Geometry: final body of the model. Coordinates: model frame, mm. Face numbers are marked on the shaded views. A direction names the side the tool comes from. Give positions to 0.01 mm unless a question says otherwise; leave off trailing zeros. Loops run counter-clockwise (first coordinate to the right, second up) from the corner with the lowest first, then second, coordinate; pieces in that order, holes last. Notation, with made-up numbers: (44.5, 19) - (80.5, 19) arc R29 cw to (80.5, 50) - close; hole circle Ø10 at (-12, 51.25). An arc over 180 degrees is marked (long way). Answer in a Markdown table with one row per item.
from build123d import *

# Parameters (mm, degrees)
BOSS_EXTRUDE1_DEPTH     = 10
CUT_EXTRUDE2_DEPTH      = 45.988887517
CUT_EXTRUDE2_DEPTH_BACK = 45.988887517
SKETCH5_R               = 2
CUT_EXTRUDE3_DEPTH      = 44.874821937


with BuildPart() as part:
    # Sketch1 → Boss-Extrude1 (new body)
    with BuildSketch(Plane.XY):
        with BuildLine():
            ThreePointArc((-15, 37.080992435), (0, 40), (15, 37.080992435))
            Line((15, 37.080992435), (15, 29.88139385))
            Line((15, 29.88139385), (3, 29.88139385))
            Line((3, 29.88139385), (3, 37.88139385))
            ThreePointArc((3, 37.88139385), (0, 38), (-3, 37.88139385))
            Line((-3, 37.88139385), (-3, 29.88139385))
            Line((-3, 29.88139385), (-15, 29.88139385))
            Line((-15, 29.88139385), (-15, 37.080992435))
        make_face()
    extrude(amount=-BOSS_EXTRUDE1_DEPTH)

    # Sketch4 → Cut-Extrude2 (cut, two sides: drawn at the far end of the back side and taken through both)
    with BuildSketch(Plane(origin=(-3, 0, 0), x_dir=(0, 0, -1), z_dir=(1, 0, 0)).offset(-CUT_EXTRUDE2_DEPTH_BACK)):
        with BuildLine():
            ThreePointArc((3, 33.88139385), (5, 31.88139385), (7, 33.88139385))
            Line((7, 33.88139385), (3, 33.88139385))
        make_face()
        with BuildLine():
            Line((3, 33.88139385), (7, 33.88139385))
            ThreePointArc((7, 33.88139385), (5, 35.88139385), (3, 33.88139385))
        make_face()
    extrude(amount=CUT_EXTRUDE2_DEPTH + CUT_EXTRUDE2_DEPTH_BACK, mode=Mode.SUBTRACT)

    # Sketch5 → Cut-Extrude3 (cut, through all)
    with BuildSketch(Plane(origin=(0, 0, 0), x_dir=(1, 0, 0), z_dir=(0, 1, 0))):
        with Locations(Location((0, 5, 0), (0, 0, 90))):
            Circle(SKETCH5_R)
    extrude(amount=CUT_EXTRUDE3_DEPTH, mode=Mode.SUBTRACT)


solid = part.part
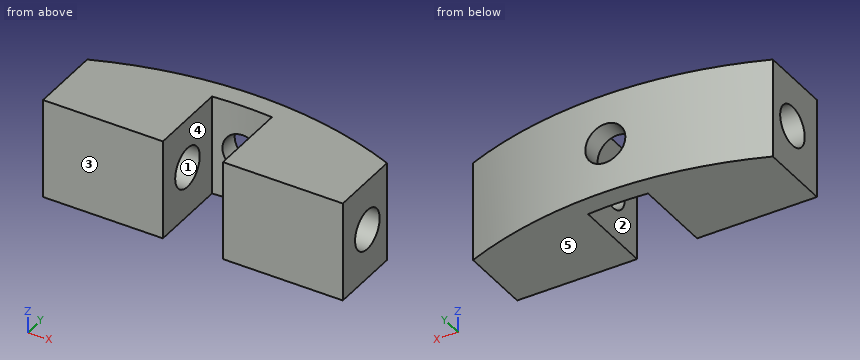
Q1. Cut plane D-D (y = 35). Output: boundary loops of the cut face in (x, z), and give its area (3 significant figures).
Check values:
| item | result |
|---|---|
| outline | (-15, -10) - (-3, -10) - (-3, -6.66) - (-15, -6.66) - close; (-15, -3.34) - (-3, -3.34) - (-3, 0) - (-15, 0) - close; (3, -10) - (15, -10) - (15, -6.66) - (3, -6.66) - close; (3, -3.34) - (15, -3.34) - (15, 0) - (3, 0) - close |
| area | 160 mm² |
Q2. Material intervals for line 1 along X through (y, z) = (36.25, -4.75); line 2 along Y through (x, z) = (10.25, -5); line 3 along Y through (x, z) = (6.5, -5), sorted ascending.
Check values:
| item | result |
|---|---|
| line 1 | -15 to -3, 3 to 15 |
| line 2 | 29.88 to 31.88, 35.88 to 38.66 |
| line 3 | 29.88 to 31.88, 35.88 to 39.47 |
Q3. Reachability of the marked faces 4 and 5 from +Z, -Z, +X, -X, +Y, -Y: full face, straight path, thin tool, end or side. Return the list, or none.
Check values:
| item | result |
|---|---|
| face 4 | +Z, -Z, -Y |
| face 5 | -Z, +X, -X, +Y, -Y |
Q4. Cut plane C-C (z = -5). Output: boundary loops of the cut face in (x, y), and give its area (3 significant figures).
Check values:
| item | result |
|---|---|
| outline | (-15, 29.88) - (-3, 29.88) - (-3, 31.88) - (-15, 31.88) - close; (-15, 35.88) - (-3, 35.88) - (-3, 37.88) arc R38 cw to (-2, 37.95) - (-2, 39.95) arc R40 ccw to (-15, 37.08) - close; (2, 37.95) arc R38 cw to (3, 37.88) - (3, 35.88) - (15, 35.88) - (15, 37.08) arc R40 ccw to (2, 39.95) - close; (3, 29.88) - (15, 29.88) - (15, 31.88) - (3, 31.88) - close |
| area | 122 mm² |
Q5. Cut plane A-A (y = 31). Output: boundary loops of the cut face in (x, z), and give its area (3 significant figures).
Check values:
| item | result |
|---|---|
| outline | (-15, -10) - (-3, -10) - (-3, 0) - (-15, 0) - close; (3, -10) - (15, -10) - (15, 0) - (3, 0) - close |
| area | 240 mm² |
Q6. Cut plane B-B (x = 0). Output: boundary loops of the cut face in (y, z), and give its area (3 significant figures).
Check values:
| item | result |
|---|---|
| outline | (38, -10) - (40, -10) - (40, -7) - (38, -7) - close; (38, -3) - (40, -3) - (40, 0) - (38, 0) - close |
| area | 12.0 mm² |
Q7. Draft query along Y for the marked faces 1, 2 and 3. Return one class per face: pulls with the +Y half, pulls with the -Y half, needs draft (parallel to the pull), parting line crosses it, or undercut.
Check values:
| item | result |
|---|---|
| face 1 | undercut |
| face 2 | needs draft |
| face 3 | pulls with the -Y half |
Q8. First-contact query: pin 1 (3 mm diameter, centred on y = 38, z = -5, fed in from -X); pin 2 (4.5 mm diameter, centred on x = 0, z = -5, fed in from -Y). Flat tips, straight axial feed; report the tip coordinate or a pass-through.
Check values:
| item | result |
|---|---|
| pin 1 | x = -15 |
| pin 2 | y = 37.93 |
